```python
from build123d import *

# Parameters (mm, degrees)
TUBO_RETANGULAR_50_X_30_X_2_6_1_DEPTH = 532
ESBO_O2_R                             = 2.5
CORTE_EXTRUS_O1_DEPTH                 = 535.554955079
ESBO_O5_R                             = 3.75
CORTE_EXTRUS_O4_DEPTH                 = 535.554955079
ESBO_O6_R                             = 3.5
CORTE_EXTRUS_O5_DEPTH                 = 535.554955079


with BuildPart() as part:
    # Sketch1 → Tubo retangular 50 X 30 X 2.6(1) (new body)
    with BuildSketch(Plane.YZ):
        with BuildLine():
            Line((-12, -25), (12, -25))
            ThreePointArc((12, -25), (14.121320344, -24.121320344), (15, -22))
            Line((15, -22), (15, 22))
            ThreePointArc((15, 22), (14.121320344, 24.121320344), (12, 25))
            Line((12, 25), (-12, 25))
            ThreePointArc((-12, 25), (-14.121320344, 24.121320344), (-15, 22))
            Line((-15, 22), (-15, -22))
            ThreePointArc((-15, -22), (-14.121320344, -24.121320344), (-12, -25))
        make_face()
        with BuildLine():
            Line((-12, -23.8), (12, -23.8))
            ThreePointArc((12, -23.8), (13.272792206, -23.272792206), (13.8, -22))
            Line((13.8, -22), (13.8, 22))
            ThreePointArc((13.8, 22), (13.272792206, 23.272792206), (12, 23.8))
            Line((12, 23.8), (-12, 23.8))
            ThreePointArc((-12, 23.8), (-13.272792206, 23.272792206), (-13.8, 22))
            Line((-13.8, 22), (-13.8, -22))
            ThreePointArc((-13.8, -22), (-13.272792206, -23.272792206), (-12, -23.8))
        make_face(mode=Mode.SUBTRACT)
    extrude(amount=TUBO_RETANGULAR_50_X_30_X_2_6_1_DEPTH)

    # Esboço2 → Corte-extrusão1 (cut, through all)
    with BuildSketch(Plane(origin=(0, 0, -25), x_dir=(-1, 0, 0), z_dir=(0, 0, -1))):
        with Locations((-58.5, 0)):
            Circle(ESBO_O2_R)
        with Locations((-33.1, 0)):
            Circle(ESBO_O2_R)
        with Locations((-7.7, 0)):
            Circle(ESBO_O2_R)
        with Locations(Location((-524.3, 0, 0), (0, 0, 180))):
            Circle(ESBO_O2_R)
        with Locations(Location((-498.9, 0, 0), (0, 0, 180))):
            Circle(ESBO_O2_R)
        with Locations(Location((-473.5, 0, 0), (0, 0, 180))):
            Circle(ESBO_O2_R)
    extrude(amount=-CORTE_EXTRUS_O1_DEPTH, mode=Mode.SUBTRACT)

    # Esboço5 → Corte-extrusão4 (cut, through all)
    with BuildSketch(Plane(origin=(0, 0, -25), x_dir=(-1, 0, 0), z_dir=(0, 0, -1))):
        with Locations((-391.484705047, 0)):
            Circle(ESBO_O5_R)
        with Locations((-142.084705047, 0)):
            Circle(ESBO_O5_R)
    extrude(amount=-CORTE_EXTRUS_O4_DEPTH, mode=Mode.SUBTRACT)

    # Esboço6 → Corte-extrusão5 (cut, through all)
    with BuildSketch(Plane(origin=(0, 0, -25), x_dir=(-1, 0, 0), z_dir=(0, 0, -1))):
        with Locations((-447.652173256, -0.984705047)):
            Circle(ESBO_O6_R)
        with Locations((-84.347826744, -0.984705047)):
            Circle(ESBO_O6_R)
    extrude(amount=-CORTE_EXTRUS_O5_DEPTH, mode=Mode.SUBTRACT)


solid = part.part
```
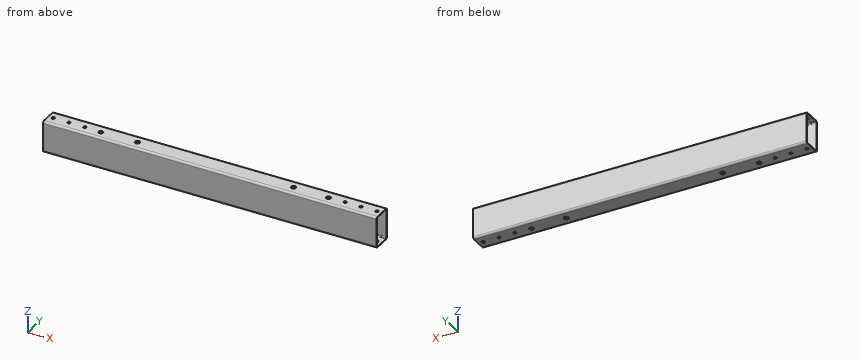
Here's how the part is built. I have some questions about the finished solid (model axes, mm). Round coordinates to 2 decimals unless told otherwise and drop trailing zeros. Order: outer loops, then holes, each group sorted by start corner. A loop starts at its lowest first (then second) coordinate and runs counter-clockwise, first axis right, second up. Notation, with made-up numbers: M 29,83 L 45,83 A16 cw 45,107 Z; hole C 77,-17.75 d7. An arc over 180 degrees is marked long. Use CSV: the item, a comma, the result in double quotes.
1) I want a section at B-B (x = 251). List the corners of the cut face in (y, z) for me, then the cut area to 3 significant figures.
Taken from the geometry:
outline,"M -15,-22 A3 ccw -12,-25 L 12,-25 A3 ccw 15,-22 L 15,22 A3 ccw 12,25 L -12,25 A3 ccw -15,22 Z; hole M -13.8,-22 A1.8 ccw -12,-23.8 L 12,-23.8 A1.8 ccw 13.8,-22 L 13.8,22 A1.8 ccw 12,23.8 L -12,23.8 A1.8 ccw -13.8,22 Z"
area,"181 mm^2"
2) I want a section at A-A (z = 14). List the corners of the cut face in (x, y) for me.
Taken from the geometry:
outline,"M 0,-15 L 532,-15 L 532,-13.8 L 0,-13.8 Z; M 0,13.8 L 532,13.8 L 532,15 L 0,15 Z"
3) I need wall thicknesses on line 1 along Y through (x, z) = (428, 3.5); line 2 along Z through (x, y) = (501.5, -4.5); line 3 along Y through (x, z) = (473.5, 24.5). Which ranges of each line are inside material? Lowest first, please. Write a range as [from, to].
Taken from the geometry:
line 1,"[-15, -13.8], [13.8, 15]"
line 2,"[-25, -23.8], [23.8, 25]"
line 3,"[-13.66, -2.5], [2.5, 13.66]"
